from build123d import *

# Parameters (mm, degrees)
BOSS_EXTRUDE1_DEPTH = 19.05
SKETCH2_R           = 38.222793673
BOSS_EXTRUDE2_DEPTH = 6.35
SKETCH3_W           = 31.75
SKETCH3_H           = 13.333086578
CUT_EXTRUDE1_DEPTH  = 6.35
SKETCH4_W           = 92.075
SKETCH4_H           = 81.28
BOSS_EXTRUDE3_DEPTH = 10.16
CHAMFER1_SIZE       = 2.54
FILLET1_R           = 1.27
SKETCH5_R           = 3.175
BOSS_EXTRUDE4_DEPTH = 15.875
BOSS_EXTRUDE5_DEPTH = 4.7625


with BuildPart() as part:
    # Sketch1 → Boss-Extrude1 (new body)
    with BuildSketch(Plane(origin=(0, 0, 0), x_dir=(0, 0, -1), z_dir=(1, 0, 0))):
        Polygon((-25.4, -5.93604562), (-25.4, 6.76395438), (0, 9.93895438), (25.4, 6.76395438), (25.4, -5.93604562), (0, -9.11104562), align=None)
    extrude(amount=-BOSS_EXTRUDE1_DEPTH)

    # Sketch2 → Boss-Extrude2 (add)
    with BuildSketch(Plane.ZY.offset(19.05)):
        with Locations(Location((0, 0, 0), (0, 0, 180))):
            Circle(SKETCH2_R)
    extrude(amount=BOSS_EXTRUDE2_DEPTH)

    # Sketch3 → Cut-Extrude1 (cut)
    with BuildSketch(Plane(origin=(-19.05, 0, 0), x_dir=(0, 0, -1), z_dir=(1, 0, 0))):
        with Locations((0, 37.6091503)):
            Rectangle(SKETCH3_W, SKETCH3_H)
    extrude(amount=-CUT_EXTRUDE1_DEPTH, mode=Mode.SUBTRACT)

    # Sketch4 → Boss-Extrude3 (add)
    with BuildSketch(Plane.ZY.offset(25.4)):
        with Locations((0, -5.869806857)):
            Rectangle(SKETCH4_W, SKETCH4_H)
    extrude(amount=BOSS_EXTRUDE3_DEPTH)

    # Chamfer1
    chamfer1_edges = [part.edges().sort_by_distance(p)[0] for p in [
        (-19.05, -38.222793673, 0),
    ]]
    chamfer(chamfer1_edges, length=CHAMFER1_SIZE)

    # Fillet1
    fillet1_edges = [part.edges().sort_by_distance(p)[0] for p in [
        (0, 0.41395438, 25.4),
        (0, 8.35145438, 12.7),
        (0, 8.35145438, -12.7),
        (0, 0.41395438, -25.4),
        (0, -7.52354562, -12.7),
        (0, -7.52354562, 12.7),
    ]]
    fillet(fillet1_edges, radius=FILLET1_R)

    # Sketch5 → Boss-Extrude4 (add)
    with BuildSketch(Plane.ZY.offset(35.56)):
        Circle(SKETCH5_R)
    extrude(amount=BOSS_EXTRUDE4_DEPTH)

    # Sketch6 → Boss-Extrude5 (add)
    with BuildSketch(Plane.ZY.offset(51.435)):
        with BuildLine():
            Line((11.624433923, 11.383749315), (7.542732602, 6.519367101))
            ThreePointArc((7.542732602, 6.519367101), (7.34328288, 4.239646347), (9.417303827, 3.272514497))
            Line((9.417303827, 3.272514497), (15.670833059, 4.375180425))
            ThreePointArc((15.670833059, 4.375180425), (17.509881849, 3.087464599), (16.222166023, 1.248415809))
            Line((16.222166023, 1.248415809), (9.968636791, 0.145749881))
            ThreePointArc((9.968636791, 0.145749881), (8.350473186, -1.472413724), (9.317605037, -3.546434671))
            Line((9.317605037, -3.546434671), (14.816866351, -6.721434671))
            ThreePointArc((14.816866351, -6.721434671), (15.397931679, -8.89), (13.229366351, -9.471065329))
            Line((13.229366351, -9.471065329), (7.730105037, -6.296065329))
            ThreePointArc((7.730105037, -6.296065329), (5.450384283, -6.49551505), (4.858095296, -8.705967643))
            Line((4.858095296, -8.705967643), (7.029923206, -14.673015785))
            ThreePointArc((7.029923206, -14.673015785), (6.081118148, -16.707734798), (4.046399135, -15.75892974))
            Line((4.046399135, -15.75892974), (1.874571225, -9.791881598))
            ThreePointArc((1.874571225, -9.791881598), (0, -8.479292695), (-1.874571225, -9.791881598))
            Line((-1.874571225, -9.791881598), (-4.046399135, -15.75892974))
            ThreePointArc((-4.046399135, -15.75892974), (-6.081118148, -16.707734798), (-7.029923206, -14.673015785))
            Line((-7.029923206, -14.673015785), (-4.858095296, -8.705967643))
            ThreePointArc((-4.858095296, -8.705967643), (-5.450384283, -6.49551505), (-7.730105037, -6.296065329))
            Line((-7.730105037, -6.296065329), (-13.229366351, -9.471065329))
            ThreePointArc((-13.229366351, -9.471065329), (-15.397931679, -8.89), (-14.816866351, -6.721434671))
            Line((-14.816866351, -6.721434671), (-9.317605037, -3.546434671))
            ThreePointArc((-9.317605037, -3.546434671), (-8.350473186, -1.472413724), (-9.968636791, 0.145749881))
            Line((-9.968636791, 0.145749881), (-16.222166023, 1.248415809))
            ThreePointArc((-16.222166023, 1.248415809), (-17.509881849, 3.087464599), (-15.670833059, 4.375180425))
            Line((-15.670833059, 4.375180425), (-9.417303827, 3.272514497))
            ThreePointArc((-9.417303827, 3.272514497), (-7.34328288, 4.239646347), (-7.542732602, 6.519367101))
            Line((-7.542732602, 6.519367101), (-11.624433923, 11.383749315))
            ThreePointArc((-11.624433923, 11.383749315), (-11.4287637, 13.620270199), (-9.192242816, 13.424599976))
            Line((-9.192242816, 13.424599976), (-5.110541495, 8.560217762))
            ThreePointArc((-5.110541495, 8.560217762), (-2.900088903, 7.967928775), (-1.5875, 9.8425))
            Line((-1.5875, 9.8425), (-1.5875, 16.1925))
            ThreePointArc((-1.5875, 16.1925), (0, 17.78), (1.5875, 16.1925))
            Line((1.5875, 16.1925), (1.5875, 9.8425))
            ThreePointArc((1.5875, 9.8425), (2.900088903, 7.967928775), (5.110541495, 8.560217762))
            Line((5.110541495, 8.560217762), (9.192242816, 13.424599976))
            ThreePointArc((9.192242816, 13.424599976), (11.4287637, 13.620270199), (11.624433923, 11.383749315))
        make_face()
    extrude(amount=BOSS_EXTRUDE5_DEPTH)


solid = part.part
Could you check a few things on this model? Use its own coordinates, in mm. A direction names the side the tool comes from. Coordinates: 2 decimals unless noted, no trailing zeros. Write each loop counter-clockwise with the first axis right and the second up, starting at its lowest first coordinate (ties: lowest second). Pieces come first, ordered by that corner, then holes. Notation, with made-up numbers: M 29.25,36 L 60.25,36 A28 ccw 60.25,69 Z; hole C 0.25,20.5 d2. An arc over 180 degrees is marked long. One line per question, with ' | ' between items.
1) For pin 1 Ø4 at (x, y) = (-53, 14.5) entering from +Z; pin 2 Ø5 at (y, z) = (-19, -3.5) entering from +X; pin 3 Ø5 at (x, y) = (-53, 12) entering from -Z, each with a flat end and sliding along its axis, tell me the tip position at first contact or that it passes through.
Checks:
pin 1: z = 11.99 | pin 2: x = -19.05 | pin 3: z = -12
2) Imagine slicing it at B-B, the plane x = -41.5. Write out the boundary of the cut face in (y, z) (3 decimals), and give its area (3 significant figures).
Checks:
outline: C 0,0 d6.35 | area: 31.7 mm²
3) I need wall thicknesses on probe 1 along X at (y, z) = (31, 36); probe 2 along X at (y, z) = (-12, -10.5); probe 3 along Y at (x, z) = (-4.5, -23). Which ranges of each line are inside material? Lowest first, please. Write a range as [from, to].
Checks:
probe 1: [-35.56, -25.4] | probe 2: [-35.56, -19.05] | probe 3: [-6.24, 7.06]
4) Imagine slicing it at A-A, the plane x = -9.5. Write out the boundary of the cut face in (y, z), and give its area (3 significant figures).
Checks:
outline: M -9.11,0 L -5.94,-25.4 L 6.76,-25.4 L 9.94,0 L 6.76,25.4 L -5.94,25.4 Z | area: 806 mm²
5) If we mould it in two halves opening along Y, with no side actions, what happens to faces 1 (the face through (-53.783, 11.026, -7.18)), 2 (the face through (-10, 0, 25.4)), 3 (the face through (-53.783, 4.269, 7.326))? For each: released by +Y, released by -Y, zero draft, split by the parting line, or undercut.
Checks:
face 1: released by +Y | face 2: zero draft | face 3: undercut
6) For faces 4 (the face through (-53.783, -1.506, -8.345)), 5 (the face through (-53.78, -11.65, 5.93)), 6 (the face through (-53.78, 7.98, 2.87)), which set-ups out of +Z, -Z, +X, -X, +Y, -Y let a thin tool reach every point of the face, with its end or its side?
Checks:
face 4: -Z, -X | face 5: -X | face 6: -X, +Y
